The drawing under review shows one solid part. Ordinate dimensions are in mm from its lowest x, y, z. A direction names the side the tool comes from. Coordinates: 2 decimals unless noted, no trailing zeros. Loops run counter-clockwise (first coordinate to the right, second up) from the corner with the lowest first, then second, coordinate; pieces in that order, holes last. Notation, with made-up numbers: M -31.5,52 L 7.5,52 A28 cw 7.5,83 Z; hole C -28,-15 d8. An arc over 180 degrees is marked long. Put each result on its own line as item: value.
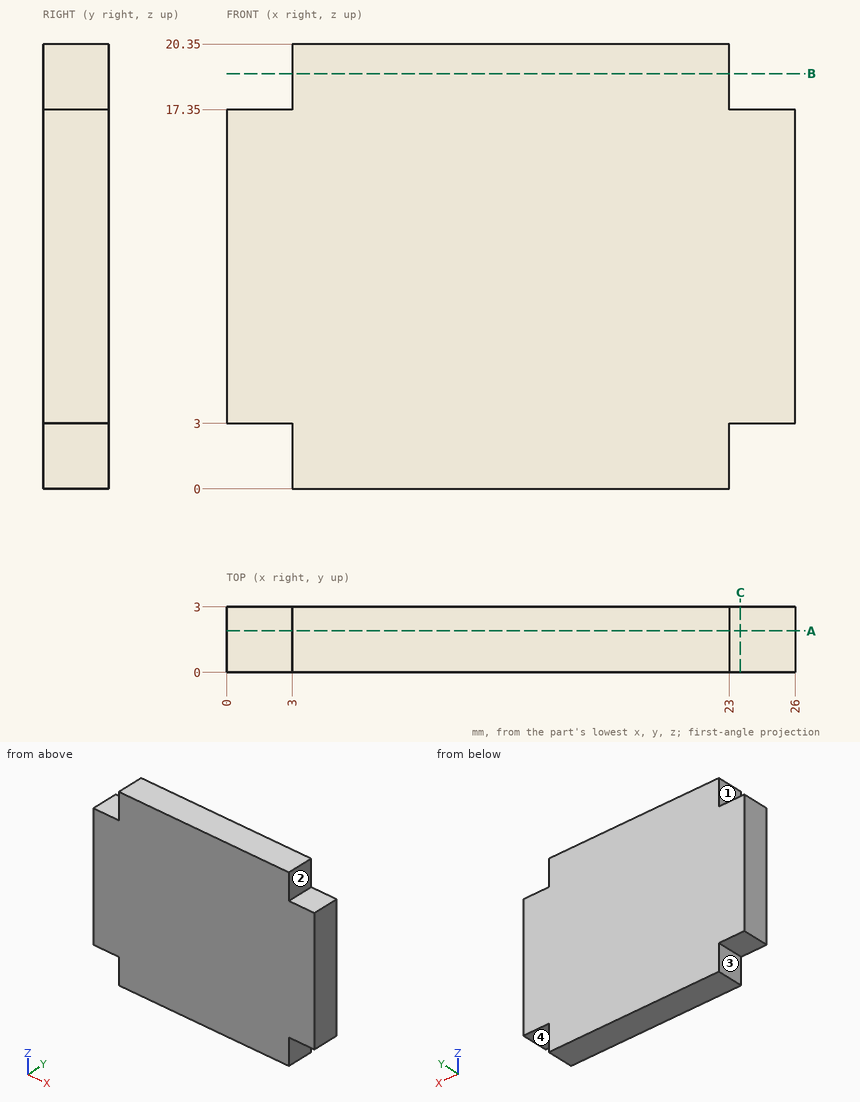
(1) For pin 1 (1.5 mm diameter, centred on y = 2, z = 18, fed in from +X); pin 2 (1.5 mm diameter, centred on x = 1.5, y = 2, fed in from -Z); pin 3 (1.5 mm diameter, centred on x = 24.5, y = 1, fed in from +Z); pin 4 (0.9 mm diameter, centred on y = 1.5, z = 1.5, fed in from +X), all flat-tipped, find the tip position at first contact; note any pin that passes through.
Determined:
pin 1: stops at x = 26
pin 2: stops at z = 3
pin 3: stops at z = 17.35
pin 4: stops at x = 23
(2) Tool access review of the marked faces 1, 2, 3 and 4: name each direction out of +Z, -Z, +X, -X, +Y, -Y from which nothing blocks a thin tool from reaching the whole face with its end or side.
Determined:
face 1: +Z, -X, +Y, -Y
face 2: +Z, +X, +Y, -Y
face 3: -Z, -X, +Y, -Y
face 4: -Z, +X, +Y, -Y
(3) Add section B-B (z = 19). Write out the cut boundary in (x, y), plus the area to 3 significant figures.
Determined:
outline: M 3,0 L 23,0 L 23,3 L 3,3 Z
area: 60.0 mm^2
(4) Add section C-C (x = 23.5). Write out the cut boundary in (y, z).
Determined:
outline: M 0,3 L 3,3 L 3,17.35 L 0,17.35 Z
(5) Wall thickness on line 1 along Z through (x, y) = (2.25, 2.45); line 2 along X through (y, z) = (0.6, 17.5): over which ranges is each line inside the solid? List them lowest first. Write a range as [from, to].
Determined:
line 1: z = [3, 17.35]
line 2: x = [3, 23]
(6) Add section A-A (y = 1.9). Write out the cut boundary in (x, z), plus the area to 3 significant figures.
Determined:
outline: M 0,3 L 3,3 L 3,0 L 23,0 L 23,3 L 26,3 L 26,17.35 L 23,17.35 L 23,20.35 L 3,20.35 L 3,17.35 L 0,17.35 Z
area: 493 mm^2
